Can you work these out from the model? Positions are in its coordinate system, mm. Round coordinates to 2 decimals unless told otherwise and drop trailing zeros.
```python
from build123d import *

# Parameters (mm, degrees)
SKETCH1_W             = 228.6
SKETCH1_H             = 254
BOSS_EXTRUDE1_DEPTH   = 6.35
F_4_40_TAPPED_HOLE1_D = 2.2606


with BuildPart() as part:
    # Sketch1 → Boss-Extrude1 (new body)
    with BuildSketch(Plane(origin=(0, 0, 0), x_dir=(1, 0, 0), z_dir=(0, 1, 0))):
        with Locations((114.3, 127)):
            Rectangle(SKETCH1_W, SKETCH1_H)
    extrude(amount=BOSS_EXTRUDE1_DEPTH)

    # #4-40 Tapped Hole1 (through all)
    with Locations(Plane(origin=(0, 6.35, 0), x_dir=(1, 0, 0), z_dir=(0, 1, 0))):
        with Locations((15.735159407, 43.18), (15.875, 58.42), (84.05884141, 57.388437181), (144.561688198, 57.388437181), (0, 127), (144.561688198, 196.611562819), (84.05884141, 196.611562819), (15.875, 195.58), (15.735159407, 210.82), (114.3, 0), (212.864840593, 43.18), (212.725, 58.42), (212.864840593, 210.82), (212.725, 195.58), (228.6, 127), (114.3, 254)):
            Hole(F_4_40_TAPPED_HOLE1_D / 2)


solid = part.part
```
(1) We'd pull the mould along Z, two halves only. Please class faces 1 (the flat face through (56, 3, -254)), 2 (the flat face through (228.6, 3, -62)), 3 (the flat face through (56, 3, 0)): released by +Z, released by -Z, zero draft, split by the parting line, or undercut.
(2) If I drill on line 1 (X direction, y = 3.5, z = -59); line 2 (X direction, y = 3, z = -195.58); line 3 (X direction, y = 6.25, z = -128), over which ranges is the centre line in solid material (lowest first)?
(3) For pin 1 (1 mm diameter, centred on x = 136, y = 2, fed in from +Z), with a flat end and sliding along its axis, tell me the tip position at first contact or that it passes through.
Check result:
1. face 1: released by -Z
1. face 2: zero draft
1. face 3: released by +Z
2. line 1: x = 0 to 14.9, 16.85 to 211.75, 213.7 to 228.6
2. line 2: x = 0 to 14.74, 17.01 to 83.6, 84.52 to 144.1, 145.02 to 211.59, 213.86 to 228.6
2. line 3: x = 0.53 to 228.07
3. pin 1: stops at z = 0
